Print and shaded views of the part. All mm, measured from the part's lowest x, y and z. A direction names the side the tool comes from. Coordinates: 2 decimals unless noted, no trailing zeros. Order: outer loops, then holes, each group sorted by start corner. A loop starts at its lowest first (then second) coordinate and runs counter-clockwise, first axis right, second up.
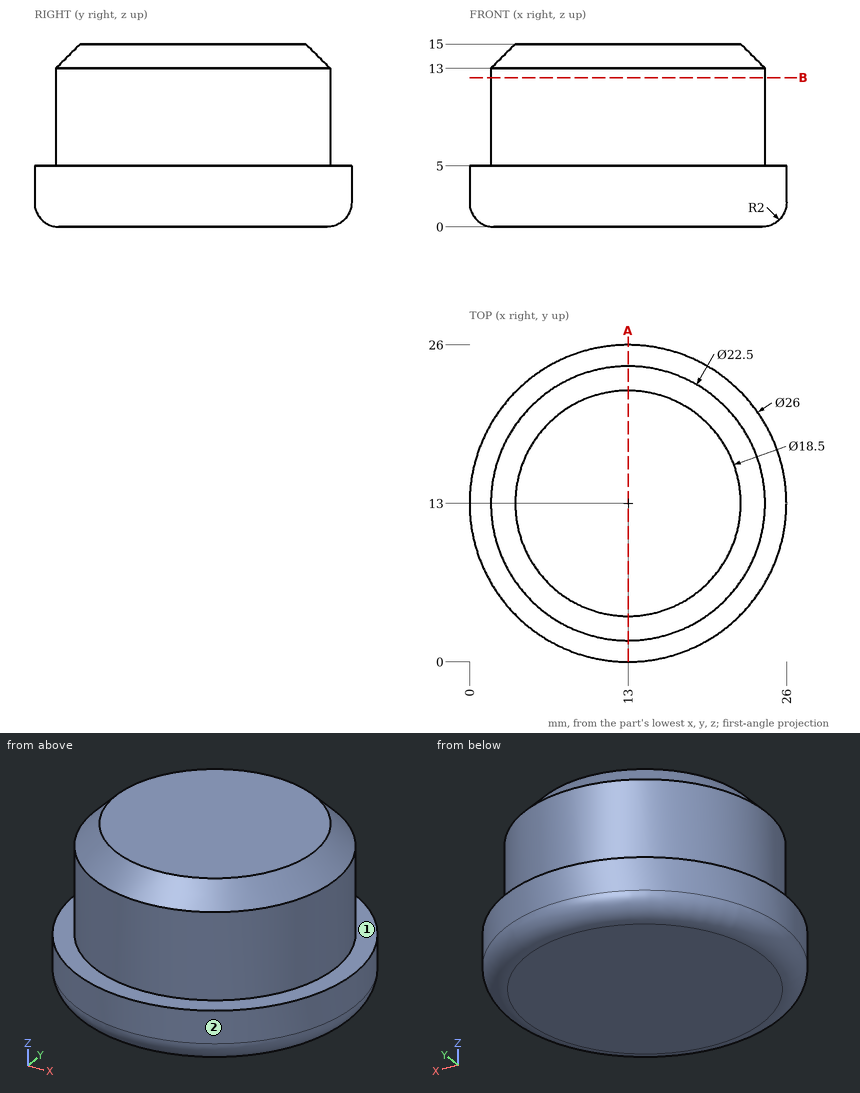
Q1. Which spindle directions (+Z, -Z, +X, -X, +Y, -Y) get a long thin tool onto all of the face, cutting with end or side? Do the marked faces 1 and 2. Say none if no direction does.
Established:
face 1: +Z
face 2: +Z, -Z
Q2. Cut at A-A, the plane x = 13. List the corners of the cut face in (y, z), plus the area to 3 significant figures.
Established:
outline: (0, 2) arc R2 ccw to (2, 0) - (24, 0) arc R2 ccw to (26, 2) - (26, 5) - (24.25, 5) - (24.25, 13) - (22.25, 15) - (3.75, 15) - (1.75, 13) - (1.75, 5) - (0, 5) - close
area: 349 mm2
Q3. Probe line 1 (Y direction, x = 12.75, z = 8); line 2 (Y direction, x = 11.25, z = 11); line 3 (X direction, y = 5, z = 6). List the from-to ranges inside material, lowest first.
Established:
line 1: y = 1.75 to 24.25
line 2: y = 1.89 to 24.11
line 3: x = 5.09 to 20.91
Q4. Cut at B-B, the plane z = 12.25. List the corners of the cut face in (x, y).
Established:
outline: circle Ø22.5 at (13, 13)
Q5. Drop flat-ended pins along their axis: P1, Ø3, axis at y = 23, z = 4.5, coming from the +X side; P2, Ø1.5, axis at x = 12.5, y = 3.5, coming from the +Z side; P3, Ø1.5, axis at y = 7, z = 11, coming from the -X side; P4, Ø5, axis at y = 16, z = 11.5, coming from the -X side. Give the stop position or say it passes through.
Established:
P1: stops at x = 22.84
P2: stops at z = 15
P3: stops at x = 3.05
P4: stops at x = 1.76
